Input: part model. Units: mm. Frame: model coordinates. A direction names the side the tool comes from. Round coordinates to 2 decimals unless told otherwise and drop trailing zeros. Write each loop counter-clockwise with the first axis right and the second up, starting at its lowest first coordinate (ties: lowest second). Pieces come first, ordered by that corner, then holes. Notation, with made-up numbers: (-34, 69) - (22, 69) arc R13 ccw to (22, 94) - close; hole circle Ø5 at (-29, 9). An arc over 180 degrees is marked (long way). Use one line per item in the form item = value.
```python
from build123d import *

# Parameters (mm, degrees)
SKETCH1_R           = 6
SKETCH1_R_2         = 6.05
SKETCH1_R_3         = 9.05
SKETCH1_R_4         = 1.05
BOSS_EXTRUDE1_DEPTH = 5
CUT_EXTRUDE1_START  = -2
CUT_EXTRUDE1_DEPTH  = 2
SKETCH3_R           = 1.25
CUT_EXTRUDE2_DEPTH  = 107.775662697


with BuildPart() as part:
    # Sketch1 → Boss-Extrude1 (new body)
    with BuildSketch(Plane.XY):
        with BuildLine():
            Line((-17.428425058, 4.5), (-24.206145914, -21.75))
            ThreePointArc((-24.206145914, -21.75), (-24.304944461, -33.854030643), (-18.705990528, -44.585714286))
            ThreePointArc((-18.705990528, -44.585714286), (-16.188386739, -51.22), (-18.705990528, -57.854285714))
            ThreePointArc((-18.705990528, -57.854285714), (-14.737892988, -94.633922608), (21.5, -87.197350822))
            Line((21.5, -87.197350822), (35.277938888, -63.977350822))
            ThreePointArc((35.277938888, -63.977350822), (38.71637128, -52.973450833), (36.851550967, -41.59667284))
            Line((36.851550967, -41.59667284), (16.613000697, 6.928795555))
            ThreePointArc((16.613000697, 6.928795555), (-1.281011782, 17.954359048), (-17.428425058, 4.5))
        make_face()
        Circle(SKETCH1_R, mode=Mode.SUBTRACT)
        with Locations((0, -28)):
            Circle(SKETCH1_R_2, mode=Mode.SUBTRACT)
        with Locations((13.777938888, -51.22)):
            Circle(SKETCH1_R_3, mode=Mode.SUBTRACT)
        with Locations((0, -74.44)):
            Circle(SKETCH1_R_3, mode=Mode.SUBTRACT)
        with Locations((0, 13)):
            Circle(SKETCH1_R_4, mode=Mode.SUBTRACT)
        with Locations((11.258330249, 6.5)):
            Circle(SKETCH1_R_4, mode=Mode.SUBTRACT)
        with Locations((11.258330249, -6.5)):
            Circle(SKETCH1_R_4, mode=Mode.SUBTRACT)
        with Locations((0, -13)):
            Circle(SKETCH1_R_4, mode=Mode.SUBTRACT)
        with Locations((-11.258330249, -6.5)):
            Circle(SKETCH1_R_4, mode=Mode.SUBTRACT)
        with Locations((-11.258330249, 6.5)):
            Circle(SKETCH1_R_4, mode=Mode.SUBTRACT)
    extrude(amount=BOSS_EXTRUDE1_DEPTH)

    # Sketch2 → Cut-Extrude1 (cut)
    with BuildSketch(Plane.XY.offset(5).offset(CUT_EXTRUDE1_START)):
        with BuildLine():
            Line((16.613000697, 6.928795555), (36.851550967, -41.59667284))
            ThreePointArc((36.851550967, -41.59667284), (38.71637128, -52.973450833), (35.277938888, -63.977350822))
            Line((35.277938888, -63.977350822), (21.5, -87.197350822))
            ThreePointArc((21.5, -87.197350822), (-14.737892988, -94.633922608), (-18.705990528, -57.854285714))
            ThreePointArc((-18.705990528, -57.854285714), (-16.188386739, -51.22), (-18.705990528, -44.585714286))
            ThreePointArc((-18.705990528, -44.585714286), (-24.304944461, -33.854030643), (-24.206145914, -21.75))
            Line((-24.206145914, -21.75), (-17.428425058, 4.5))
            ThreePointArc((-17.428425058, 4.5), (-1.281011782, 17.954359048), (16.613000697, 6.928795555))
        make_face()
        with BuildLine():
            Line((9.468285508, 9.39955156), (5.467787499, 2.470485754))
            ThreePointArc((5.467787499, 2.470485754), (3, 5.196152423), (-0.594390327, 5.970485754))
            Line((-0.594390327, 5.970485754), (3.406107682, 12.89955156))
            ThreePointArc((3.406107682, 12.89955156), (3.46289335, 14.794014563), (1.913207856, 15.885201783))
            ThreePointArc((1.913207856, 15.885201783), (-9.022746373, 13.213252737), (-15.491933385, 4))
            Line((-15.491933385, 4), (-22.269654241, -22.25))
            ThreePointArc((-22.269654241, -22.25), (-20.946970822, -37.498653241), (-10.347792006, -48.540769231))
            ThreePointArc((-10.347792006, -48.540769231), (-8.697504007, -51.22), (-10.347792006, -53.899230769))
            ThreePointArc((-10.347792006, -53.899230769), (-16.813726675, -90.133903125), (19.78, -86.176762756))
            Line((19.78, -86.176762756), (21.416047429, -83.419527323))
            ThreePointArc((21.416047429, -83.419527323), (22.868749584, -79.189380689), (22.517294907, -74.730573258))
            ThreePointArc((22.517294907, -74.730573258), (22.927957655, -72.188598464), (25.15802624, -70.901324657))
            ThreePointArc((25.15802624, -70.901324657), (28.527716294, -69.789192601), (31.009004018, -67.252490018))
            Line((31.009004018, -67.252490018), (33.557938888, -62.956762756))
            ThreePointArc((33.557938888, -62.956762756), (36.721296689, -52.833174766), (35.005662001, -42.366539013))
            Line((35.005662001, -42.366539013), (24.369440107, -16.864334436))
            ThreePointArc((24.369440107, -16.864334436), (22.811532345, -15.020784633), (20.47666212, -14.409120101))
            ThreePointArc((20.47666212, -14.409120101), (17.701744194, -12.866781789), (17.865596008, -9.696272437))
            ThreePointArc((17.865596008, -9.696272437), (19.084800596, -6.438585473), (18.585469893, -2.996252973))
            Line((18.585469893, -2.996252973), (14.76711173, 6.158929383))
            ThreePointArc((14.76711173, 6.158929383), (13.890682857, 7.940335621), (12.800384361, 9.599487498))
            ThreePointArc((12.800384361, 9.599487498), (11.080545761, 10.395960893), (9.468285508, 9.39955156))
        make_face(mode=Mode.SUBTRACT)
    extrude(amount=CUT_EXTRUDE1_DEPTH, mode=Mode.SUBTRACT)

    # Sketch3 → Cut-Extrude2 (cut, through all)
    with BuildSketch(Plane.XY.offset(3)):
        with Locations((20.325912078, -11.412910091)):
            Circle(SKETCH3_R)
        with Locations((-11.697504007, -51.22)):
            Circle(SKETCH3_R)
        with Locations((25.397635129, -73.891740611)):
            Circle(SKETCH3_R)
    extrude(amount=-CUT_EXTRUDE2_DEPTH, mode=Mode.SUBTRACT)


solid = part.part
```
(1) Cut plane A-A on y = -51.22. Output: boundary loops of the cut face in (x, z), then the cut area to 3 significant figures.
Derived:
outline = (-16.19, 0) - (-12.95, 0) - (-12.95, 3) - (-16.19, 3) - close; (-10.45, 0) - (4.73, 0) - (4.73, 5) - (-8.7, 5) - (-8.7, 3) - (-10.45, 3) - close; (22.83, 0) - (38.78, 0) - (38.78, 3) - (36.78, 3) - (36.78, 5) - (22.83, 5) - close
area = 158 mm^2
(2) Access query for faces 1 (the face through (16.7, 1.52, 3.99)), 2 (the face through (-18.833, -8.941, 3.986)), 3 (the face through (1.38, 9.39, 3.99)), 4 (the face through (22.907, -72.219, 3.986)), 5 (the face through (-0.79, -22, 2.46)). Directions: +Z, -Z, +X, -X, +Y, -Y. A direction counts if a zero-diameter tool reaches every point of the face in a straight line with its end or side. Return the directions, or none.
Derived:
face_1 = +Z, +X, +Y
face_2 = +Z, -X, +Y
face_3 = +Z
face_4 = +Z, +X
face_5 = +Z, -Z
(3) Cut plane D-D on y = -28. Output: boundary loops of the cut face in (x, z), then the cut area to 3 significant figures.
Derived:
outline = (-25, 0) - (-6.05, 0) - (-6.05, 5) - (-23, 5) - (-23, 3) - (-25, 3) - close; (6.05, 0) - (31.18, 0) - (31.18, 3) - (29.01, 3) - (29.01, 5) - (6.05, 5) - close
area = 212 mm^2
(4) Cut plane B-B on z = 1.3. Count the separate pieces of the cut face and the enclosed holes in it, then the cut area to 3 significant figures.
Derived:
separate_pieces = 1
enclosed_holes = 13
area = 4,700 mm^2
(5) Cut plane C-C on y = 0. Output: boundary loops of the cut face in (x, z).
Derived:
outline = (-18.59, 0) - (-6, 0) - (-6, 5) - (-16.52, 5) - (-16.52, 3) - (-18.59, 3) - close; (6, 0) - (19.5, 0) - (19.5, 3) - (17.34, 3) - (17.34, 5) - (6, 5) - close
(6) First-contact query: pin 1 Ø12 at (x, y) = (18, -69) entering from -Z; pin 2 Ø4 at (x, y) = (-11.7, -51.22) entering from +Z; pin 3 Ø3 at (y, z) = (-71, 2) entering from +X. Flat tips, straight axial feed; report the tip coordinate or a pass-through.
Derived:
pin_1 = 0
pin_2 = 3
pin_3 = 32
(7) Draft query along Y for faces 6 (the face through (22, -55, 2)), 7 (the face through (28.485, -69.816, 3.986)), 8 (the face through (29.76, -29.79, 3.99)). Return one class per face: released by +Y, released by -Y, zero draft, split by the parting line, or undercut.
Derived:
face_6 = undercut
face_7 = released by -Y
face_8 = released by +Y
(8) Material intervals for L1, parallel to Y at x = 0, z = 1; L2, parallel to Y at x = 7.5, z = 4.65; L3, parallel to Y at x = 11.5, z = 4.4, sorted ascending.
Derived:
L1 = -99.44 to -83.49, -65.39 to -34.05, -21.95 to -14.05, -11.95 to -6, 6 to 11.95, 14.05 to 18
L2 = -96.18 to -79.5, -69.38 to -57.74, -44.7 to 5.99
L3 = -94.36 to -59.98, -42.46 to -7.52, -5.48 to 5.48, 7.52 to 10.38
